Check sheet for the modelled part. Datum: model origin and axes. Units: mm. A direction names the side the tool comes from. Give positions to 0.01 mm unless a question says otherwise; leave off trailing zeros. Loops run counter-clockwise (first coordinate to the right, second up) from the corner with the lowest first, then second, coordinate; pieces in that order, holes last. Notation, with made-up numbers: (-6.5, 62) - (-0.5, 62) arc R27 ccw to (-0.5, 80) - close; hole circle Ø7 at (38, -14). An arc over 180 degrees is marked (long way). Use CSV: the item, a comma, the result in double quotes.
from build123d import *

# Parameters (mm, degrees)
SKETCH2_R           = 9.6012
SKETCH2_R_2         = 2.4892
SKETCH2_R_3         = 3.2639
SKETCH2_R_4         = 11.1252
SKETCH2_R_5         = 14.3002
SKETCH2_R_6         = 2.413
BOSS_EXTRUDE1_DEPTH = 6.35
SKETCH3_R           = 3.2639
SKETCH3_R_2         = 2.413
SKETCH3_R_3         = 2.4892
CUT_EXTRUDE1_DEPTH  = 177.630627937


with BuildPart() as part:
    # Sketch2 → Boss-Extrude1 (new body)
    with BuildSketch(Plane(origin=(0, 0, 0), x_dir=(1, 0, 0), z_dir=(0, 1, 0))):
        Polygon((-155.087712155, 84.29625), (-89.463193808, -29.36875), (82.46904885, -29.36875), (82.46904885, 84.29625), align=None)
        with Locations(Location((-41.275, 2.38125, 0), (0, 0, 270))):
            Circle(SKETCH2_R, mode=Mode.SUBTRACT)
        with Locations(Location((-41.275, 27.78125, 0), (0, 0, 270))):
            Circle(SKETCH2_R_2, mode=Mode.SUBTRACT)
        with Locations(Location((-41.275, -23.01875, 0), (0, 0, 270))):
            Circle(SKETCH2_R_2, mode=Mode.SUBTRACT)
        with Locations(Location((-82.130845389, -16.66875, 0), (0, 0, 270))):
            Circle(SKETCH2_R_3, mode=Mode.SUBTRACT)
        with Locations(Location((-133.090666899, 71.59625, 0), (0, 0, 270))):
            Circle(SKETCH2_R_3, mode=Mode.SUBTRACT)
        with Locations(Location((-5.496024757, 21.654924548, 0), (0, 0, 270))):
            Circle(SKETCH2_R_4, mode=Mode.SUBTRACT)
        with Locations(Location((32.48383617, 1.11125, 0), (0, 0, 270))):
            Circle(SKETCH2_R_5, mode=Mode.SUBTRACT)
        with Locations(Location((61.774869917, 67.406835627, 0), (0, 0, 270))):
            Circle(SKETCH2_R_6, mode=Mode.SUBTRACT)
        with Locations(Location((76.11904885, -23.01875, 0), (0, 0, 270))):
            Circle(SKETCH2_R_3, mode=Mode.SUBTRACT)
    extrude(amount=BOSS_EXTRUDE1_DEPTH)

    # Sketch3 → Cut-Extrude1 (cut, through all)
    # profile 1 of 18: a face of its own
    with BuildSketch(Plane(origin=(0, 6.35, 0), x_dir=(1, 0, 0), z_dir=(0, 1, 0))):
        with BuildLine():
            Line((-50.704696238, 58.032833483), (-112.240521983, 73.58273966))
            Line((-112.240521983, 73.58273966), (-81.745655831, 20.764082115))
            ThreePointArc((-81.745655831, 20.764082115), (-66.664634619, 38.866438144), (-44.45, 46.717712139))
            Line((-44.45, 46.717712139), (-44.45, 50.396621207))
            ThreePointArc((-44.45, 50.396621207), (-48.64368552, 53.341307868), (-50.704696238, 58.032833483))
        make_face()
    # profile 2 of 18: a face of its own
    with BuildSketch(Plane(origin=(0, 6.35, 0), x_dir=(1, 0, 0), z_dir=(0, 1, 0))):
        with BuildLine():
            Line((-38.1, 50.396621207), (-38.1, 46.717712139))
            ThreePointArc((-38.1, 46.717712139), (-25.920369141, 44.095010454), (-14.947020834, 38.195213939))
            ThreePointArc((-14.947020834, 38.195213939), (-11.907888955, 39.593444485), (-8.671024757, 40.438477859))
            Line((-8.671024757, 40.438477859), (-8.671024757, 54.678493879))
            ThreePointArc((-8.671024757, 54.678493879), (-11.283169826, 56.093396277), (-13.332375749, 58.244211411))
            Line((-13.332375749, 58.244211411), (-32.382270315, 55.964402602))
            ThreePointArc((-32.382270315, 55.964402602), (-34.629883571, 52.552798441), (-38.1, 50.396621207))
        make_face()
    # profile 3 of 18: a face of its own
    with BuildSketch(Plane(origin=(0, 6.35, 0), x_dir=(1, 0, 0), z_dir=(0, 1, 0))):
        with BuildLine():
            ThreePointArc((-133.733764479, 62.092984745), (-142.13305739, 68.602790594), (-139.277335877, 78.838539138))
            Line((-139.277335877, 78.838539138), (-132.888385663, 84.29625))
            Line((-132.888385663, 84.29625), (-155.087712155, 84.29625))
            Line((-155.087712155, 84.29625), (-89.463193808, -29.36875))
            Line((-89.463193808, -29.36875), (-60.133800133, -29.36875))
            Line((-60.133800133, -29.36875), (-83.452466562, -26.101615019))
            ThreePointArc((-83.452466562, -26.101615019), (-91.274629988, -19.336488408), (-88.317514367, -9.426460862))
            Line((-88.317514367, -9.426460862), (-77.153529536, 0.110286058))
            Line((-77.153529536, 0.110286058), (-112.093783272, 60.628580757))
            Line((-112.093783272, 60.628580757), (-133.733764479, 62.092984745))
        make_face()
    # profile 4 of 18: a face of its own
    with BuildSketch(Plane(origin=(0, 6.35, 0), x_dir=(1, 0, 0), z_dir=(0, 1, 0))):
        Polygon((82.46904885, 84.29625), (-132.888385663, 84.29625), (51.53383617, 84.100664467), (51.53383617, -29.36875), (82.46904885, -29.36875), align=None)
        with Locations((76.11904885, -23.01875)):
            Circle(SKETCH3_R, mode=Mode.SUBTRACT)
        with Locations((61.774869917, 67.406835627)):
            Circle(SKETCH3_R_2, mode=Mode.SUBTRACT)
    # profile 5 of 18: a face of its own
    with BuildSketch(Plane(origin=(0, 6.35, 0), x_dir=(1, 0, 0), z_dir=(0, 1, 0))):
        with BuildLine():
            Line((45.18383617, 15.310281657), (45.18383617, 77.94625))
            Line((45.18383617, 77.94625), (41.398231111, 77.94625))
            ThreePointArc((41.398231111, 77.94625), (41.117229303, 70.57627228), (35.65883617, 65.616284578))
            Line((35.65883617, 65.616284578), (35.65883617, 19.894803311))
            ThreePointArc((35.65883617, 19.894803311), (40.745698306, 18.276451253), (45.18383617, 15.310281657))
        make_face()
    # profile 6 of 18: a face of its own
    with BuildSketch(Plane(origin=(0, 6.35, 0), x_dir=(1, 0, 0), z_dir=(0, 1, 0))):
        with BuildLine():
            Line((-44.45, 77.94625), (-103.5894656, 77.94625))
            Line((-103.5894656, 77.94625), (-49.449869194, 64.2653473))
            ThreePointArc((-49.449869194, 64.2653473), (-47.307458964, 66.748109508), (-44.45, 68.357133449))
            Line((-44.45, 68.357133449), (-44.45, 77.94625))
        make_face()
    # profile 7 of 18: a face of its own
    with BuildSketch(Plane(origin=(0, 6.35, 0), x_dir=(1, 0, 0), z_dir=(0, 1, 0))):
        with BuildLine():
            Line((-8.671024757, 77.94625), (-38.1, 77.94625))
            Line((-38.1, 77.94625), (-38.1, 68.357133449))
            ThreePointArc((-38.1, 68.357133449), (-35.487854931, 66.942231051), (-33.438649008, 64.791415916))
            Line((-33.438649008, 64.791415916), (-14.388754442, 67.071224726))
            ThreePointArc((-14.388754442, 67.071224726), (-12.141141186, 70.482828886), (-8.671024757, 72.639006121))
            Line((-8.671024757, 72.639006121), (-8.671024757, 77.94625))
        make_face()
    # profile 8 of 18: a face of its own
    with BuildSketch(Plane(origin=(0, 6.35, 0), x_dir=(1, 0, 0), z_dir=(0, 1, 0))):
        with BuildLine():
            Line((-2.321024757, 54.678493879), (-2.321024757, 40.438477859))
            ThreePointArc((-2.321024757, 40.438477859), (0.074866406, 39.872160113), (2.377715421, 39.001587501))
            Line((2.377715421, 39.001587501), (22.15801549, 68.318685604))
            Line((22.15801549, 68.318685604), (4.01215469, 63.092933247))
            ThreePointArc((4.01215469, 63.092933247), (2.114261551, 57.93082129), (-2.321024757, 54.678493879))
        make_face()
    # profile 9 of 18: a face of its own
    with BuildSketch(Plane(origin=(0, 6.35, 0), x_dir=(1, 0, 0), z_dir=(0, 1, 0))):
        with BuildLine():
            ThreePointArc((7.641632189, 35.450013166), (13.004757083, 26.196242782), (12.536001856, 15.510942435))
            Line((12.536001856, 15.510942435), (17.472938166, 12.840505779))
            ThreePointArc((17.472938166, 12.840505779), (22.730759734, 17.475234846), (29.30883617, 19.894803311))
            Line((29.30883617, 19.894803311), (29.30883617, 65.614932157))
            ThreePointArc((29.30883617, 65.614932157), (28.790391012, 65.815305481), (28.284516096, 66.045577972))
            Line((28.284516096, 66.045577972), (7.641632189, 35.450013166))
        make_face()
    # profile 10 of 18: a face of its own
    with BuildSketch(Plane(origin=(0, 6.35, 0), x_dir=(1, 0, 0), z_dir=(0, 1, 0))):
        with BuildLine():
            Line((14.451809556, 7.255232113), (9.514873246, 9.925668769))
            ThreePointArc((9.514873246, 9.925668769), (6.605195221, 6.942243792), (3.116401587, 4.662908409))
            ThreePointArc((3.116401587, 4.662908409), (3.08719182, -0.411318161), (2.479854635, -5.449152025))
            ThreePointArc((2.479854635, -5.449152025), (8.985543719, -4.351211356), (15.13161349, -6.750230017))
            ThreePointArc((15.13161349, -6.750230017), (13.456237349, 0.187679153), (14.451809556, 7.255232113))
        make_face()
    # profile 11 of 18: a face of its own
    with BuildSketch(Plane(origin=(0, 6.35, 0), x_dir=(1, 0, 0), z_dir=(0, 1, 0))):
        with BuildLine():
            ThreePointArc((-38.1, 60.133460575), (-41.275, 62.640777328), (-44.45, 60.133460575))
            Line((-44.45, 60.133460575), (-44.45, 58.62029408))
            ThreePointArc((-44.45, 58.62029408), (-41.275, 56.112977328), (-38.1, 58.62029408))
            Line((-38.1, 58.62029408), (-38.1, 60.133460575))
        make_face()
    # profile 12 of 18: a face of its own
    with BuildSketch(Plane(origin=(0, 6.35, 0), x_dir=(1, 0, 0), z_dir=(0, 1, 0))):
        with BuildLine():
            ThreePointArc((-2.321024757, 72.639006121), (0.231903953, 71.269036308), (2.254864024, 69.194935338))
            Line((2.254864024, 69.194935338), (22.97374411, 75.161681012))
            ThreePointArc((22.97374411, 75.161681012), (23.165063227, 76.576202255), (23.565616004, 77.94625))
            Line((23.565616004, 77.94625), (-2.321024757, 77.94625))
            Line((-2.321024757, 77.94625), (-2.321024757, 72.639006121))
        make_face()
    # profile 13 of 18: a face of its own
    with BuildSketch(Plane(origin=(0, 6.35, 0), x_dir=(1, 0, 0), z_dir=(0, 1, 0))):
        with BuildLine():
            Line((18.349161012, -23.01875), (45.18383617, -23.01875))
            Line((45.18383617, -23.01875), (45.18383617, -13.087781657))
            ThreePointArc((45.18383617, -13.087781657), (32.282698959, -17.937688128), (19.486846811, -12.816447857))
            ThreePointArc((19.486846811, -12.816447857), (20.025058188, -18.04104949), (18.349161012, -23.01875))
        make_face()
    # profile 14 of 18: a face of its own
    with BuildSketch(Plane(origin=(0, 6.35, 0), x_dir=(1, 0, 0), z_dir=(0, 1, 0))):
        with Locations(Location((32.481923558, 74.59586426, 0), (0, 0, 270))):
            Circle(SKETCH3_R)
    # profile 15 of 18: a face of its own
    with BuildSketch(Plane(origin=(0, 6.35, 0), x_dir=(1, 0, 0), z_dir=(0, 1, 0))):
        with Locations(Location((-5.496024757, 63.65875, 0), (0, 0, 270))):
            Circle(SKETCH3_R)
    # profile 16 of 18: a face of its own
    with BuildSketch(Plane(origin=(0, 6.35, 0), x_dir=(1, 0, 0), z_dir=(0, 1, 0))):
        with Locations(Location((7.71883617, -16.66875, 0), (0, 0, 270))):
            Circle(SKETCH3_R)
    # profile 17 of 18: a face of its own
    with BuildSketch(Plane(origin=(0, 6.35, 0), x_dir=(1, 0, 0), z_dir=(0, 1, 0))):
        with Locations(Location((-5.496024757, 36.386924548, 0), (0, 0, 270))):
            Circle(SKETCH3_R_3)
    # profile 18 of 18: a face of its own
    with BuildSketch(Plane(origin=(0, 6.35, 0), x_dir=(1, 0, 0), z_dir=(0, 1, 0))):
        with Locations(Location((-5.496024757, 6.922924548, 0), (0, 0, 270))):
            Circle(SKETCH3_R_3)
    extrude(amount=-CUT_EXTRUDE1_DEPTH, mode=Mode.SUBTRACT)


solid = part.part
1. Sectioned sample at A-A, the plane z = 2. Record the boundary of the cut face in (x, y).
Completed:
outline,"(-79.62, 0) - (-49.82, 0) - (-49.82, 6.35) - (-79.62, 6.35) - close; (-32.73, 0) - (2.96, 0) - (2.96, 6.35) - (-32.73, 6.35) - close; (13.69, 0) - (18.53, 0) - (18.53, 6.35) - (13.69, 6.35) - close; (46.44, 0) - (51.53, 0) - (51.53, 6.35) - (46.44, 6.35) - close"
2. Sectioned sample at D-D, the plane x = -27. Record the boundary of the cut face in (y, z), and give its area (3 significant figures).
Completed:
outline,"(0, -84.18) - (6.35, -84.18) - (6.35, -77.95) - (0, -77.95) - close; (0, -65.56) - (6.35, -65.56) - (6.35, -56.61) - (0, -56.61) - close; (0, -44.48) - (6.35, -44.48) - (6.35, 29.37) - (0, 29.37) - close"
area,"565 mm²"
3. Set-up check for faces 1 (the face through (-82.81, 3.22, 4.72)), 2 (the face through (-8.671, 3, -47)): record each of +Z, -Z, +X, -X, +Y, -Y from which the full face is reachable in a straight line by a thin tool's end or side.
Completed:
face 1,"-X, +Y, -Y"
face 2,"+Y, -Y"
4. Scan lines: line 1 along X through (y, z) = (4.25, -1.5); line 2 along X through (y, z) = (2.5, -43.5); line 3 along X through (y, z) = (3, -37). Record each from-to range of solid material in increasing order.
Completed:
line 1,"x = -77.96 to -50.84, -31.71 to 3.17, 13.44 to 18.19, 46.78 to 51.53"
line 2,"x = -102.2 to -94.87, -58.16 to -24.39, -8.67 to -2.32, 5.41 to 13.07, 29.31 to 35.66, 45.18 to 51.53"
line 3,"x = -98.45 to -91.12, -69.16 to -7.91, -3.08 to 8.69, 29.31 to 35.66, 45.18 to 51.53"
5. Sectioned sample at C-C, the plane z = -23. Record the boundary of the cut face in (x, y).
Completed:
outline,"(-90.37, 0) - (-83.04, 0) - (-83.04, 6.35) - (-90.37, 6.35) - close; (-80.65, 0) - (-16.54, 0) - (-16.54, 6.35) - (-80.65, 6.35) - close; (5.55, 0) - (13.51, 0) - (13.51, 6.35) - (5.55, 6.35) - close; (29.31, 0) - (35.66, 0) - (35.66, 6.35) - (29.31, 6.35) - close; (45.18, 0) - (51.53, 0) - (51.53, 6.35) - (45.18, 6.35) - close"
6. Sectioned sample at B-B, the plane x = -95.5. Record the boundary of the cut face in (y, z).
Completed:
outline,"(0, -84.26) - (6.35, -84.26) - (6.35, -77.95) - (0, -77.95) - close; (0, -75.9) - (6.35, -75.9) - (6.35, -69.35) - (0, -69.35) - close; (0, -44.59) - (6.35, -44.59) - (6.35, -31.89) - (0, -31.89) - close"
7. Release check for a two-part mould opening along Z. For faces 3 (the face through (-136.128, 3.219, -81.529)), 4 (the face through (-8.671, 3, -75)) record: released by +Z, released by -Z, zero draft, split by the parting line, or undercut.
Completed:
face 3,"released by -Z"
face 4,"undercut"
8. Go/stop test with flat-tipped pins: pin 1 Ø3 at (y, z) = (4.5, -73.5) entering from -X; pin 2 Ø1.9 at (y, z) = (3, -45) entering from -X. Record where each tip stops, or that it passes through.
Completed:
pin 1,"stops at x = -142.61"
pin 2,"stops at x = -103.62"
